Geometry check sheet. Reference: the model listing, model coordinates, mm. A direction names the side the tool comes from. Give positions to 0.01 mm unless a question says otherwise; leave off trailing zeros. Order: outer loops, then holes, each group sorted by start corner. A loop starts at its lowest first (then second) coordinate and runs counter-clockwise, first axis right, second up.
Autodesk Inventor part; units mm, degrees
ref_plane "YZ Plane" through (0, 0, 0) normal (1, 0, 0) x (0, 1, 0)
ref_plane "XZ Plane" through (0, 0, 0) normal (0, 1, 0) x (-1, 0, 0)
ref_plane "XY Plane" through (0, 0, 0) normal (0, 0, 1) x (1, 0, 0)
sketch "Sketch1" plane through (0, 0, 0) normal (0, 0, 1) x (1, 0, 0)
  circle A0 centre (0, 0) radius 25
  circle A1 centre (0, 0) radius 100
  circle A2 centre (0, 0) radius 30
  dimension "d0" = 50
  dimension "d1" = 200
  dimension "d2" = 5
extrude "Extrusion1" add sketch "Sketch1" along normal blind 3.7 contours A1 | A2
move or copy body "Move Body1" bodies to move or copy 1 copy no translate (0, 0, 50)
mirror "Mirror1" about plane through (0, 0, 0) normal (0, 0, 1)
extrude "Extrusion2" add sketch "Sketch1" against normal up to surface (107.4 mm away) from surface at 53.7 contours A2
properties part number "roll" material "Plywood, Finish"
Item 1: Sectioned sample at C-C (z = -26.5). Enter the section's corners in (x, y).
Reported:
outline: circle Ø60 at (0, 0); hole circle Ø50 at (0, 0)
Item 2: Scan lines: L1, parallel to Y at x = 0, z = 25; L2, parallel to Z at x = 69.5, y = 67; L3, parallel to Y at x = -16, z = 19. Record each from-to range of solid material in increasing order.
Reported:
L1: y = -30 to -25, 25 to 30
L2: z = -53.7 to -50, 50 to 53.7
L3: y = -25.38 to -19.21, 19.21 to 25.38
Item 3: Gauge pin test, flat ends, axial feed: pin 1 (8 mm diameter, centred on x = -68.5, y = -79.5, fed in from -Z); pin 2 (1 mm diameter, centred on y = -12, z = 36.5, fed in from +X). Record the tip position at first contact, or that the pin passes through.
Reported:
pin 1: passes through
pin 2: stops at x = 27.71
Item 4: Sectioned sample at D-D (x = 76.5). Enter the section's corners in (y, z).
Reported:
outline: (-64.4, -53.7) - (64.4, -53.7) - (64.4, -50) - (-64.4, -50) - close; (-64.4, 50) - (64.4, 50) - (64.4, 53.7) - (-64.4, 53.7) - close
Item 5: Draft check along Z on faces 3 (the flat face through (-21, -21, -53.7)), 4 (the cylindrical face through (-29.97, 1.32, 0.7)), 5 (the flat face through (21, -21, 53.7)), 6 (the cylindrical face through (95.38, 30.04, -51.82)). Enter one of: released by +Z, released by -Z, zero draft, split by the parting line, or undercut.
Reported:
face 3: released by -Z
face 4: undercut
face 5: released by +Z
face 6: zero draft
Item 6: Sectioned sample at A-A (x = 0). Enter the section's corners in (y, z), and give its area (3 significant figures).
Reported:
outline: (-100, -53.7) - (-25, -53.7) - (-25, 53.7) - (-100, 53.7) - (-100, 50) - (-30, 50) - (-30, -50) - (-100, -50) - close; (25, -53.7) - (100, -53.7) - (100, -50) - (30, -50) - (30, 50) - (100, 50) - (100, 53.7) - (25, 53.7) - close
area: 2,110 mm2
Item 7: Set-up check for faces 1 (the cylindrical face through (95.38, -30.04, 51.82)), 2 (the flat face through (21, 24, 50)): record each of +Z, -Z, +X, -X, +Y, -Y from which the full face is reachable in a straight line by a thin tool's end or side.
Reported:
face 1: +Z, -Z
face 2: none
